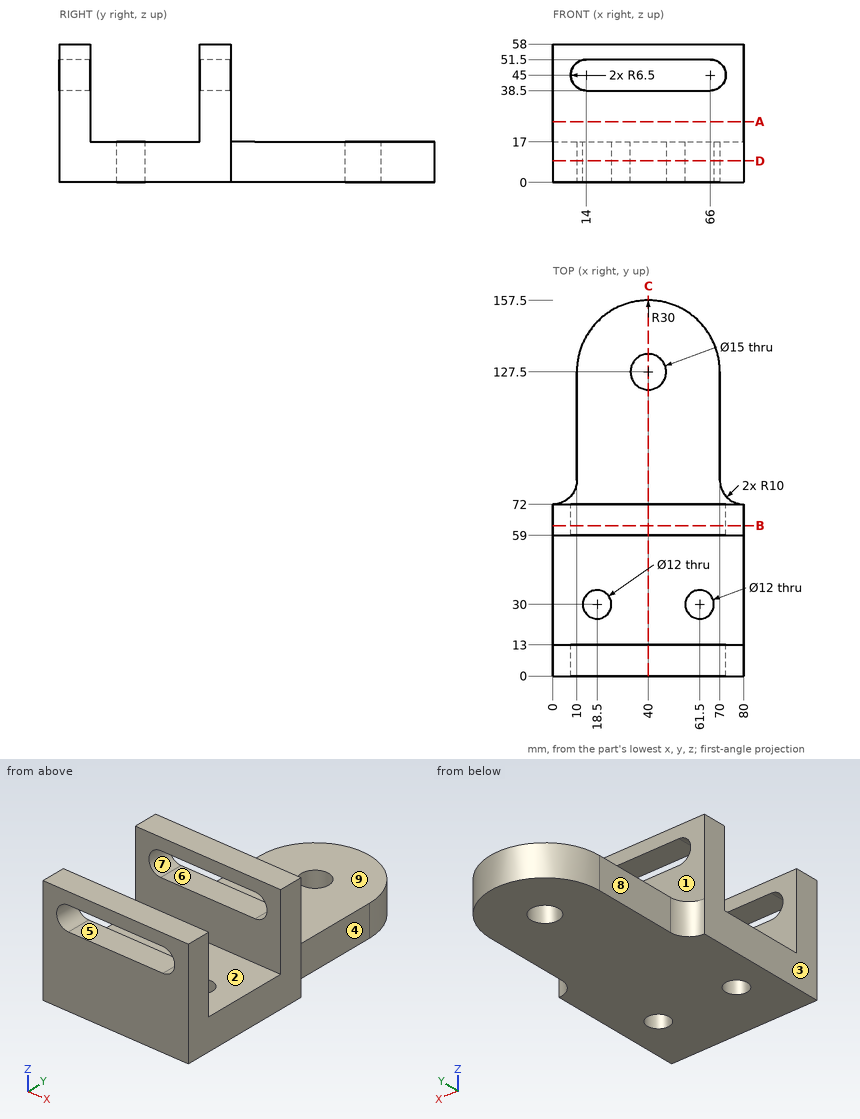
Verification items for this drawing (mm, ordinates from the low corner). A direction names the side the tool comes from. Give positions to 0.01 mm unless a question says otherwise; leave off trailing zeros. Order: outer loops, then holes, each group sorted by start corner. A loop starts at its lowest first (then second) coordinate and runs counter-clockwise, first axis right, second up.
1) Gauge pin test, flat ends, axial feed: pin 1 (10 mm diameter, centred on x = 28, z = 10, fed in from +Y); pin 2 (4 mm diameter, centred on x = 10, z = 19.5, fed in from +Y); pin 3 (8.5 mm diameter, centred on y = 100.5, z = 9.5, fed in from -X); pin 4 (7 mm diameter, centred on x = 61.5, y = 30, fed in from +Z). Record the tip position at first contact, or that the pin passes through.
Results are:
pin 1: stops at y = 156.67
pin 2: stops at y = 72
pin 3: stops at x = 10
pin 4: passes through
2) Draft check along X on the marked faces 6, 7, 8 and 9. Enter one of: released by +X, released by -X, zero draft, split by the parting line, or undercut.
Results are:
face 6: undercut
face 7: undercut
face 8: released by -X
face 9: zero draft
3) Cross-section at C-C (x = 40). Record the boundary of the cut face in (y, z), then the cut area to 3 significant figures.
Results are:
outline: (0, 0) - (120, 0) - (120, 17) - (72, 17) - (72, 38.5) - (59, 38.5) - (59, 17) - (13, 17) - (13, 38.5) - (0, 38.5) - close; (0, 51.5) - (13, 51.5) - (13, 58) - (0, 58) - close; (59, 51.5) - (72, 51.5) - (72, 58) - (59, 58) - close; (135, 0) - (157.5, 0) - (157.5, 17) - (135, 17) - close
area: 3,150 mm2
4) Cross-section at B-B (y = 63). Record the boundary of the cut face in (x, z).
Results are:
outline: (0, 0) - (80, 0) - (80, 58) - (0, 58) - close; hole (14, 38.5) - (66, 38.5) arc R6.5 ccw to (66, 51.5) - (14, 51.5) arc R6.5 ccw to start
5) Cross-section at D-D (z = 9). Give the number of separate pieces and of enclosed holes in the cut face, then the cut area to 3 significant figures.
Results are:
separate pieces: 1
enclosed holes: 3
area: 10,100 mm2
6) Tool access check on the marked faces 1, 2, 3, 4 and 5. Record the directions out of +Z, -Z, +X, -X, +Y, -Y that give a thin tool (end or side, any length) a straight path to the whole face; none if there is none.
Results are:
face 1: +Z, +X, -X, +Y
face 2: +Z, +X, -X
face 3: +Z, -Z, -X, +Y, -Y
face 4: +Z, -Z, +X, +Y
face 5: +Y, -Y
7) Material ranges on probe 1 along Z at (x, y) = (65, 62); probe 2 along Y at (x, z) = (16, 24.5); probe 3 along Y at (x, z) = (40, 10.25), recorded low to high.
Results are:
probe 1: z = 0 to 38.5, 51.5 to 58
probe 2: y = 0 to 13, 59 to 72
probe 3: y = 0 to 120, 135 to 157.5
8) Cross-section at A-A (z = 25.5). Record the boundary of the cut face in (x, y).
Results are:
outline: (0, 0) - (80, 0) - (80, 13) - (0, 13) - close; (0, 59) - (80, 59) - (80, 72) - (0, 72) - close
